```python
from build123d import *

# Parameters (mm, degrees)
F0_W          = 115
F0_H          = 50
F1_DEPTH      = 3
F1_DEPTH_BACK = 3
F2_R          = 5
F2_R_2        = 1.2
F2_R_3        = 1.5
F3_DEPTH      = 6.001
F4_R          = 1.2
F5_DEPTH      = 5.1471356602
F6_R          = 1.2
F7_DEPTH      = 10


with BuildPart() as f1:
    # F0 (on Front) → F1 (new body, two sides)
    with BuildSketch(Plane.XZ) as f1_sk:
        Rectangle(F0_W, F0_H)
    extrude(amount=F1_DEPTH)
    extrude(f1_sk.sketch, amount=-F1_DEPTH_BACK)

    # F2 (on face) → F3 (cut, through all)
    with BuildSketch(Plane.XZ.offset(3)):
        with Locations((49.5, 15)):
            Circle(F2_R)
        with Locations((-37.5, 22)):
            Circle(F2_R_2)
        with Locations((-27.5, 22)):
            Circle(F2_R_2)
        with Locations((-32.5, 15)):
            Circle(F2_R_3)
        with Locations((-37.5, 8)):
            Circle(F2_R_2)
        with Locations((-44.5, 8)):
            Circle(F2_R_2)
    extrude(amount=-F3_DEPTH, mode=Mode.SUBTRACT)

    # F4 (on face) → F5 (cut, through all)
    with BuildSketch(Plane.XY.offset(25)):
        with Locations((49.5, 0)):
            Circle(F4_R)
    extrude(amount=-F5_DEPTH, mode=Mode.SUBTRACT)

    # F6 (on face) → F7 (cut)
    with BuildSketch(Plane(origin=(0, 0, -25), x_dir=(1, 0, 0), z_dir=(0, 0, -1))):
        with Locations((-40, 0)):
            Circle(F6_R)
        with Locations((40, 0)):
            Circle(F6_R)
    extrude(amount=-F7_DEPTH, mode=Mode.SUBTRACT)


solid = f1.part
```
Here's how the part is built. I have some questions about the finished solid (model axes, mm). A direction names the side the tool comes from. Coordinates: 2 decimals unless noted, no trailing zeros. Write each loop counter-clockwise with the first axis right and the second up, starting at its lowest first coordinate (ties: lowest second). Pieces come first, ordered by that corner, then holes. Notation, with made-up numbers: M 77,37 L 111,37 A30 cw 111,59 Z; hole C 54.25,-37.5 d6. An arc over 180 degrees is marked long. Answer as CSV lines item,"result". Start each with the question number.
Q1. Suppose I cut it at B-B, the plane x = -27.5. List the corners of the cut face in (y, z) for me, then the cut area to 3 significant figures.
Q2. Suppose I cut it at A-A, the plane z = 22. List the corners of the cut face in (x, y) for me.
Q3. Suppose I cut it at D-D, the plane y = 0. List the corners of the cut face in (x, z) for me, then the cut area to 3 significant figures.
Q4. Suppose I cut it at C-C, the plane z = 15. List the corners of the cut face in (x, y) for me.
Q5. I need wall thicknesses on probe 1 along X at (y, z) = (0, -23); probe 2 along Z at (x, y) = (-27.5, 1.65); probe 3 along Z at (x, y) = (-37.5, -0.35). Which ranges of each line are inside material? Lowest first, please. Write a range as [from, to].
Q6. For faces 1 (the flat face through (40, 0, -15)), 2 (the cylindrical face through (-43.39, -0.04, 7.54)), which set-ups out of +Z, -Z, +X, -X, +Y, -Y let a thin tool reach every point of the face, with its end or its side?
Q7. If we mould it in two halves opening along Z, with no side actions, what happens to faces 3 (the cylindrical face through (-33.7, 0, 14.1)), 4 (the cylindrical face through (50.61, -0.46, 22.46)), 5 (the cylindrical face through (-36.39, -0.04, 7.54)), 6 (the flat face through (-1, 0, 25))? For each: pulls with the +Z half, pulls with the -Z half, needs draft (parallel to the pull), parting line crosses it, or undercut.
Q8. Will this pin go through, and if not, where does the flat tip stop? pin 1 Ø1.9 at (x, y) = (-40, 0) entering from -Z.
Entries:
1,outline,"M -3,-25 L 3,-25 L 3,20.8 L -3,20.8 Z; M -3,23.2 L 3,23.2 L 3,25 L -3,25 Z"
1,area,"286 mm²"
2,outline,"M -57.5,-3 L -38.7,-3 L -38.7,3 L -57.5,3 Z; M -36.3,-3 L -28.7,-3 L -28.7,3 L -36.3,3 Z; M -26.3,-3 L 57.5,-3 L 57.5,3 L -26.3,3 Z; hole C 49.5,0 d2.4"
3,outline,"M -57.5,-25 L -41.2,-25 L -41.2,-15 L -38.8,-15 L -38.8,-25 L 38.8,-25 L 38.8,-15 L 41.2,-15 L 41.2,-25 L 57.5,-25 L 57.5,25 L 50.7,25 L 50.7,19.85 A5 cw long 48.3,19.85 L 48.3,25 L -57.5,25 Z; hole C -44.5,8 d2.4; hole C -37.5,8 d2.4; hole C -37.5,22 d2.4; hole C -32.5,15 d3; hole C -27.5,22 d2.4"
3,area,"5,590 mm²"
4,outline,"M -57.5,-3 L -34,-3 L -34,3 L -57.5,3 Z; M -31,-3 L 44.5,-3 L 44.5,3 L -31,3 Z; M 54.5,-3 L 57.5,-3 L 57.5,3 L 54.5,3 Z"
5,probe 1,"x = [-57.5, -41.2], [-38.8, 38.8], [41.2, 57.5]"
5,probe 2,"z = [-25, 20.8], [23.2, 25]"
5,probe 3,"z = [-25, 6.8], [9.2, 20.8], [23.2, 25]"
6,face 1,"-Z"
6,face 2,"+Y, -Y"
7,face 3,"undercut"
7,face 4,"needs draft"
7,face 5,"undercut"
7,face 6,"pulls with the +Z half"
8,pin 1,"stops at z = -15"
